Here's how the part is built. I have some questions about the finished solid (model axes, mm). Face numbers are marked on the shaded views. A direction names the side the tool comes from. Coordinates: 2 decimals unless noted, no trailing zeros. Write each loop counter-clockwise with the first axis right and the second up, starting at its lowest first coordinate (ties: lowest second). Pieces come first, ordered by that corner, then holes.
Item 1: We'd pull the mould along Z, two halves only. Please class the marked faces 1, 2, 3 and 4: +Z half, -Z half, draft (parallel to the pull), parting line (faces both ways), or undercut.
Item 2: For the marked faces 5, 6, 7, 8 and 9, which set-ups out of +Z, -Z, +X, -X, +Y, -Y let a thin tool reach every point of the face, with its end or its side?
Item 3: If I drill on line 1 (X direction, y = 8, z = 13); line 2 (X direction, y = 52, z = 18); line 3 (Y direction, x = -20, z = 26.5) (3 decimals), over which ranges is the centre line in solid material (lowest first)?
Item 4: If we section it at B-B (z = -16): Please give me the cut outline in (x, y), then the cut area to 3 significant figures.
Item 5: I'm going to push flat-ended pins straight in: pin 1 Ø10 at (x, z) = (-26, -14.5) entering from +Y; pin 2 Ø6 at (x, z) = (38.5, -9.5) entering from -Y; pin 3 Ø2.5 at (x, z) = (31.5, -4.5) entering from -Y; pin 4 Ø1.4 at (x, y) = (-40.5, 4.5) entering from -Z. Where does each tip first touch, or does it pass through?
Item 6: If we section it at C-C (y = 22): Please give me the cut outline in (x, z) (3 decimals), then the cut area to 3 significant figures.
Item 7: If we section it at A-A (x = 12.5): Please give me the cut outline in (y, z) (3 decimals), then the cut area to 3 significant figures.
Item 8: If we section it at D-D (z = 27.5): Please give me the cut outline in (x, y) (3 decimals).
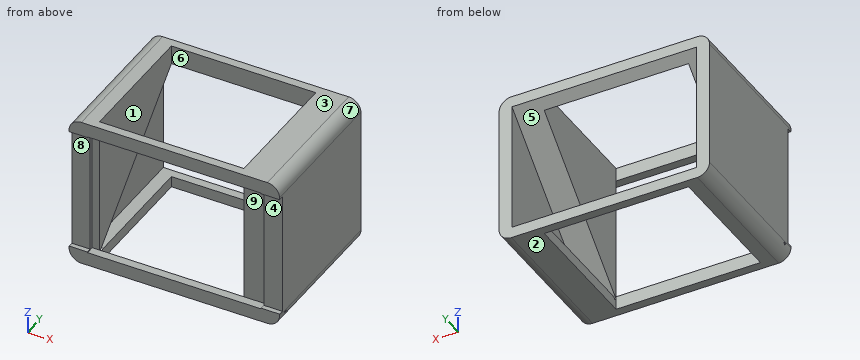
from build123d import *

# Parameters (mm, degrees)
SKETCH_1_W               = 86
SKETCH_1_H               = 62
SKETCH_1_W_2             = 71
SKETCH_1_H_2             = 51
EXTRUDE_1_DEPTH          = 60
SKETCH_2_W               = 75.5
SKETCH_2_H               = 53.03
CUT_EXTRUDE_1_DEPTH      = 56.5
EXTRUDE_2_DEPTH          = 76
SKETCH_4_W               = 59
SKETCH_4_H               = 53.03
CUT_EXTRUDE_2_DEPTH      = 97.400207469
CUT_EXTRUDE_3_DEPTH      = 97.908461963
CUT_EXTRUDE_3_DEPTH_BACK = 97.908461963
SKETCH_7_W               = 86
SKETCH_7_H               = 50.4
CUT_EXTRUDE_4_DEPTH      = 2
FILLET_1_R               = 5
FILLET_2_R               = 3


with BuildPart() as part:
    # 草图1 → 凸台-拉伸1 (new body)
    with BuildSketch(Plane(origin=(0, 0, 0), x_dir=(1, 0, 0), z_dir=(0, 1, 0))):
        Rectangle(SKETCH_1_W, SKETCH_1_H)
        Rectangle(SKETCH_1_W_2, SKETCH_1_H_2, mode=Mode.SUBTRACT)
    extrude(amount=EXTRUDE_1_DEPTH)

    # 草图2 → 切除-拉伸1 (cut)
    with BuildSketch(Plane(origin=(0, 60, 0), x_dir=(1, 0, 0), z_dir=(0, 1, 0))):
        Rectangle(SKETCH_2_W, SKETCH_2_H)
    extrude(amount=-CUT_EXTRUDE_1_DEPTH, mode=Mode.SUBTRACT)

    # 草图3 → 凸台-拉伸2 (add)
    with BuildSketch(Plane(origin=(-37.75, 0, 0), x_dir=(0, 0, -1), z_dir=(1, 0, 0))):
        Polygon((26.515, 3.5), (-26.515, 60), (-26.515, 3.5), align=None)
    extrude(amount=EXTRUDE_2_DEPTH)

    # 草图4 → 切除-拉伸2 (cut, through all)
    with BuildSketch(Plane.XY.offset(31)):
        with Locations((-3, 30)):
            Rectangle(SKETCH_4_W, SKETCH_4_H)
    extrude(amount=-CUT_EXTRUDE_2_DEPTH, mode=Mode.SUBTRACT)

    # 草图5 → 切除-拉伸3 (cut, two sides: drawn at the far end of the back side and taken through both)
    with BuildSketch(Plane.ZY.offset(-26.5).offset(-CUT_EXTRUDE_3_DEPTH_BACK)):
        Polygon((-26.515, 3.5), (-27.363528137, 4.348528137), (-26.515, 5.197056275), align=None)
    extrude(amount=CUT_EXTRUDE_3_DEPTH + CUT_EXTRUDE_3_DEPTH_BACK, mode=Mode.SUBTRACT)

    # 草图7 → 切除-拉伸4 (cut)
    with BuildSketch(Plane.XZ):
        Rectangle(SKETCH_7_W, SKETCH_7_H)
    extrude(amount=-CUT_EXTRUDE_4_DEPTH, mode=Mode.SUBTRACT)

    # 圆角1
    # the kernel refuses this fillet: 5 mm, written as the material it takes off along each edge
    with BuildSketch(Plane(origin=(43, -12.5, 31), x_dir=(-1, 0, 0), z_dir=(0, 1, 0)), Plane(origin=(43, -12.5, -31), x_dir=(0, 0, 1), z_dir=(0, 1, 0))) as fillet_1_piece_1:
        with BuildLine():
            CenterArc((FILLET_1_R, -FILLET_1_R), FILLET_1_R, 90, 90)
            Line((0, -FILLET_1_R), (0, 0))
            Line((0, 0), (FILLET_1_R, 0))
        make_face()
    extrude(amount=85, mode=Mode.SUBTRACT)
    with BuildSketch(Plane(origin=(-43, -12.5, 31), x_dir=(1, 0, 0), z_dir=(0, 1, 0)), Plane(origin=(-43, -12.5, -31), x_dir=(0, 0, 1), z_dir=(0, 1, 0))) as fillet_1_piece_2:
        with BuildLine():
            CenterArc((FILLET_1_R, FILLET_1_R), FILLET_1_R, 180, 90)
            Line((0, FILLET_1_R), (0, 0))
            Line((0, 0), (FILLET_1_R, 0))
        make_face()
    extrude(amount=85, mode=Mode.SUBTRACT)

    # 圆角2
    # the kernel refuses this fillet: 3 mm, written as the material it takes off along each edge
    with BuildSketch(Plane(origin=(37.75, 5.197056275, -26.515), x_dir=(0, 1, 0), z_dir=(-1, 0, 0))) as fillet_2_piece_1_section:
        with BuildLine():
            CenterArc((FILLET_2_R * 0.414213562373, FILLET_2_R), FILLET_2_R, 225, 45)
            Line((-FILLET_2_R * 0.292893218813, FILLET_2_R * 0.292893218813), (0, 0))
            Line((0, 0), (FILLET_2_R * 0.414213562373, 0))
        make_face()
    fillet_2_piece_1 = extrude(amount=14.356601718, mode=Mode.PRIVATE)
    fillet_2_piece_1 = split(fillet_2_piece_1, bisect_by=Plane(origin=(32.125, 4.476160676, -27.491160676), z_dir=(0, 0.7071067811865434, 0.7071067811865518)), keep=Keep.TOP, mode=Mode.PRIVATE)
    add(fillet_2_piece_1, mode=Mode.SUBTRACT)
    with BuildSketch(Plane(origin=(-29.393398282, 5.197056275, -26.515), x_dir=(0, 1, 0), z_dir=(-1, 0, 0))) as fillet_2_piece_2_section:
        with BuildLine():
            CenterArc((FILLET_2_R * 0.414213562373, FILLET_2_R), FILLET_2_R, 225, 45)
            Line((-FILLET_2_R * 0.292893218813, FILLET_2_R * 0.292893218813), (0, 0))
            Line((0, 0), (FILLET_2_R * 0.414213562373, 0))
        make_face()
    fillet_2_piece_2 = extrude(amount=8.356601718, mode=Mode.PRIVATE)
    fillet_2_piece_2 = split(fillet_2_piece_2, bisect_by=Plane(origin=(-35.125, 4.476160676, -27.491160676), z_dir=(0, 0.7071067811865434, 0.7071067811865518)), keep=Keep.TOP, mode=Mode.PRIVATE)
    add(fillet_2_piece_2, mode=Mode.SUBTRACT)


solid = part.part
Answer list:
1. face 1: draft
1. face 2: -Z half
1. face 3: +Z half
1. face 4: undercut
2. face 5: +Y
2. face 6: +Z, -Z
2. face 7: +Z, +X, +Y, -Y
2. face 8: +X, -X, -Y
2. face 9: -Y
3. line 1: x = -43 to -32.5, 26.5 to 43
3. line 2: x = -43 to -37.75, 37.75 to 43
3. line 3: y = 0 to 3.485, 56.515 to 59.984
4. outline: (-43, 2) - (-35.5, 2) - (-35.5, 3.5) - (-32.5, 3.5) - (-32.5, 14.7) - (-37.75, 14.7) - (-37.75, 60) - (-43, 60) - close; (26.5, 3.5) - (35.5, 3.5) - (35.5, 2) - (43, 2) - (43, 60) - (37.75, 60) - (37.75, 14.7) - (26.5, 14.7) - close
4. area: 801 mm2
5. pin 1: passes through
5. pin 2: stops at y = 2
5. pin 3: stops at y = 3.5
5. pin 4: stops at z = -30.66
6. outline: (-43, -26) arc R5 ccw to (-38, -31) - (-32.5, -31) - (-32.5, -26.515) - (-37.75, -26.515) - (-37.75, -9.151) - (-32.5, -9.151) - (-32.5, 31) - (-38, 31) arc R5 ccw to (-43, 26) - close; (26.5, -31) - (38, -31) arc R5 ccw to (43, -26) - (43, 26) arc R5 ccw to (38, 31) - (26.5, 31) - (26.5, -9.151) - (37.75, -9.151) - (37.75, -26.515) - (26.5, -26.515) - close
6. area: 1,370 mm2
7. outline: (0, -31) - (3.485, -31) - (3.485, -25.5) - (0, -25.5) - close; (0, 25.5) - (3.485, 25.5) - (3.485, 31) - (0, 31) - close; (56.515, -31) - (60, -31) - (60, -26.515) - (56.515, -26.515) - close; (56.515, 23.244) - (60, 26.515) - (60, 31) - (56.515, 31) - close
7. area: 75.3 mm2
8. outline: (-42.77, 0) - (42.77, 0) - (42.77, 60) - (-42.77, 60) - close; hole (-32.5, 3.485) - (26.5, 3.485) - (26.5, 56.515) - (-32.5, 56.515) - close
